For this review, take the finished solid that the model builds, in its own axes (mm). Face numbers are marked on the shaded views. Give positions to 0.01 mm unless a question says otherwise; leave off trailing zeros. Order: outer loops, then holes, each group sorted by start corner. A loop starts at its lowest first (then second) coordinate and runs counter-clockwise, first axis right, second up. Notation, with made-up numbers: (88, -9) - (98, -9) arc R27 cw to (98, 19) - close; hole circle Ø2 at (-39.75, 39.5). An arc over 180 degrees is marked (long way). One line per item, written item: value.
```python
from build123d import *

# Parameters (mm, degrees)
BASE_FLANGE1_OUTLINE_W       = 203.2
BASE_FLANGE1_OUTLINE_H       = 3.175
BASE_FLANGE1_DEPTH           = 101.6
EDGE_FLANGE1_STRIP_W         = 14.1732
EDGE_FLANGE1_STRIP_H         = 3.175
EDGE_FLANGE1_STRIP_CUT_DEPTH = 101.6
EDGE_FLANGE1_DEPTH           = 101.6
EDGE_FLANGE2_STRIP_W         = 14.1732
EDGE_FLANGE2_STRIP_H         = 3.175
EDGE_FLANGE2_STRIP_CUT_DEPTH = 101.6
EDGE_FLANGE2_DEPTH           = 101.6
SKETCH38_R                   = 3.175
CUT_EXTRUDE2_DEPTH           = 229.6
SKETCH45_R                   = 3.175
CUT_EXTRUDE3_DEPTH           = 12.7


# Read off the part's stored shape, not the designer's step: Base-Flange1
# Sheet-metal steps are written as plain solids
with BuildPart() as part:
    # Base-Flange1 outline → Base-Flange1 (new body)
    with BuildSketch(Plane.XY):
        with Locations((-101.6, 1.5875)):
            Rectangle(BASE_FLANGE1_OUTLINE_W, BASE_FLANGE1_OUTLINE_H)
    extrude(amount=BASE_FLANGE1_DEPTH)

    # Edge-Flange1 strip (across the edge) → Edge-Flange1 strip cut (cut)
    with BuildSketch(Plane(origin=(-203.2, 3.175, 0), x_dir=(1, 0, 0), z_dir=(0, 0, 1))):
        with Locations((-3.175, -1.5875)):
            Rectangle(EDGE_FLANGE1_STRIP_W, EDGE_FLANGE1_STRIP_H)
    extrude(amount=EDGE_FLANGE1_STRIP_CUT_DEPTH, mode=Mode.SUBTRACT)

    # Edge-Flange1 section (across the edge) → Edge-Flange1 (add)
    with BuildSketch(Plane(origin=(-203.2, 3.175, 0), x_dir=(1, 0, 0), z_dir=(0, 0, 1))):
        with BuildLine():
            Line((0, 0.7366), (0, 22.225))
            Line((0, 22.225), (3.175, 22.225))
            Line((3.175, 22.225), (3.175, 0.7366))
            ThreePointArc((3.175, 0.7366), (3.390745145, 0.215745145), (3.9116, 0))
            Line((3.9116, 0), (3.9116, -3.175))
            ThreePointArc((3.9116, -3.175), (1.145681115, -2.029318885), (0, 0.7366))
        make_face()
    extrude(amount=EDGE_FLANGE1_DEPTH)

    # Edge-Flange2 strip (across the edge) → Edge-Flange2 strip cut (cut)
    with BuildSketch(Plane(origin=(0, 3.175, 101.6), x_dir=(-1, 0, 0), z_dir=(0, 0, -1))):
        with Locations((-3.175, -1.5875)):
            Rectangle(EDGE_FLANGE2_STRIP_W, EDGE_FLANGE2_STRIP_H)
    extrude(amount=EDGE_FLANGE2_STRIP_CUT_DEPTH, mode=Mode.SUBTRACT)

    # Edge-Flange2 section (across the edge) → Edge-Flange2 (add)
    with BuildSketch(Plane(origin=(0, 3.175, 101.6), x_dir=(-1, 0, 0), z_dir=(0, 0, -1))):
        with BuildLine():
            Line((0, 0.7366), (0, 22.225))
            Line((0, 22.225), (3.175, 22.225))
            Line((3.175, 22.225), (3.175, 0.7366))
            ThreePointArc((3.175, 0.7366), (3.390745145, 0.215745145), (3.9116, 0))
            Line((3.9116, 0), (3.9116, -3.175))
            ThreePointArc((3.9116, -3.175), (1.145681115, -2.029318885), (0, 0.7366))
        make_face()
    extrude(amount=EDGE_FLANGE2_DEPTH)

    # Sketch38 → Cut-Extrude2 (cut, through all)
    with BuildSketch(Plane(origin=(0, 0, 0), x_dir=(0, 0, -1), z_dir=(1, 0, 0))):
        with Locations(Location((-12.7, 12.7, 0), (0, 0, 90))):
            Circle(SKETCH38_R)
        with Locations(Location((-88.9, 12.7, 0), (0, 0, 90))):
            Circle(SKETCH38_R)
    extrude(amount=-CUT_EXTRUDE2_DEPTH, mode=Mode.SUBTRACT)

    # Sketch45 → Cut-Extrude3 (cut)
    with BuildSketch(Plane(origin=(0, 3.175, 0), x_dir=(1, 0, 0), z_dir=(0, 1, 0))):
        with Locations(Location((-177.8, -50.8, 0), (0, 0, 270))):
            Circle(SKETCH45_R)
        with Locations(Location((-25.4, -50.8, 0), (0, 0, 270))):
            Circle(SKETCH45_R)
    extrude(amount=-CUT_EXTRUDE3_DEPTH, mode=Mode.SUBTRACT)


solid = part.part
```
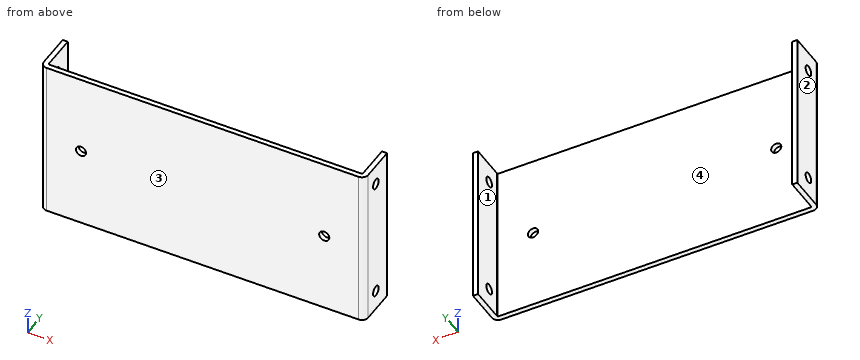
(1) For P1, Ø1, axis at x = -143.5, z = 90, coming from the +Y side (3 decimals), flat-tipped, find the tip position at first contact; note if it passes through.
Answers below:
P1: stops at y = 3.175
(2) Take a section at D-D (z = 77). Write out the cut boundary in (x, y) (3 decimals), then the cut area to 3 significant figures.
Answers below:
outline: (-203.2, 3.912) arc R3.912 ccw to (-199.288, 0) - (-3.912, 0) arc R3.912 ccw to (0, 3.912) - (0, 25.4) - (-3.175, 25.4) - (-3.175, 3.912) arc R0.737 cw to (-3.912, 3.175) - (-199.288, 3.175) arc R0.737 cw to (-200.025, 3.912) - (-200.025, 25.4) - (-203.2, 25.4) - close
area: 780 mm^2
(3) Draft analysis for pull direction X (two halves, no side actions). For the marked faces 1, 2, 3 and 4, state which applies: pulls with the +X half, pulls with the -X half, needs draft (parallel to the pull), parting line crosses it, or undercut.
Answers below:
face 1: undercut
face 2: pulls with the -X half
face 3: needs draft
face 4: undercut
(4) Take a section at A-A (y = 12.7). Write out the cut boundary in (x, z) (3 decimals).
Answers below:
outline: (-203.2, 0) - (-200.025, 0) - (-200.025, 9.525) - (-203.2, 9.525) - close; (-203.2, 15.875) - (-200.025, 15.875) - (-200.025, 85.725) - (-203.2, 85.725) - close; (-203.2, 92.075) - (-200.025, 92.075) - (-200.025, 101.6) - (-203.2, 101.6) - close; (-3.175, 0) - (0, 0) - (0, 9.525) - (-3.175, 9.525) - close; (-3.175, 15.875) - (0, 15.875) - (0, 85.725) - (-3.175, 85.725) - close; (-3.175, 92.075) - (0, 92.075) - (0, 101.6) - (-3.175, 101.6) - close
(5) Take a section at C-C (x = -177.8). Write out the cut boundary in (y, z) (3 decimals).
Answers below:
outline: (0, 0) - (3.175, 0) - (3.175, 47.625) - (0, 47.625) - close; (0, 53.975) - (3.175, 53.975) - (3.175, 101.6) - (0, 101.6) - close
(6) Wall thickness on line 1 (Z direction, x = -201.55, y = 12.7) (3 decimals); line 2 (X direction, y = 11.5, z = 76) (3 decimals); line 3 (Z direction, x = -177.8, y = 1.2) (3 decimals): over which ranges is each line inside the solid? List them lowest first. Write a range as from..to.
Answers below:
line 1: z = 0..9.525, 15.875..85.725, 92.075..101.6
line 2: x = -203.2..-200.025, -3.175..0
line 3: z = 0..47.625, 53.975..101.6
(7) Take a section at B-B (z = 50.8). Write out the cut boundary in (x, y) (3 decimals), then the cut area to 3 significant figures.
Answers below:
outline: (-203.2, 3.912) arc R3.912 ccw to (-199.288, 0) - (-180.975, 0) - (-180.975, 3.175) - (-199.288, 3.175) arc R0.737 cw to (-200.025, 3.912) - (-200.025, 25.4) - (-203.2, 25.4) - close; (-174.625, 0) - (-28.575, 0) - (-28.575, 3.175) - (-174.625, 3.175) - close; (-22.225, 0) - (-3.912, 0) arc R3.912 ccw to (0, 3.912) - (0, 25.4) - (-3.175, 25.4) - (-3.175, 3.912) arc R0.737 cw to (-3.912, 3.175) - (-22.225, 3.175) - close
area: 740 mm^2
